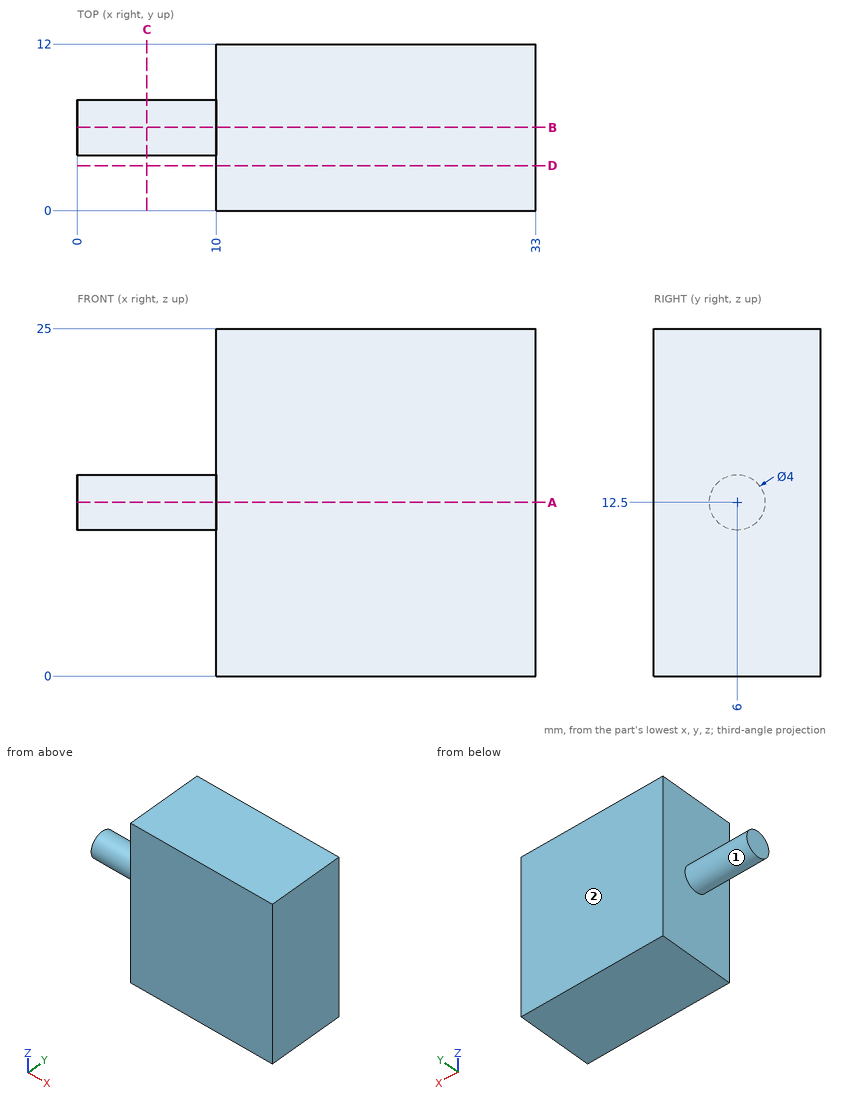
Geometry: see drawing. Coordinates: mm, zero at the bounding-box minimum. A direction names the side the tool comes from. Round coordinates to 2 decimals unless told otherwise and drop trailing zeros. Write each loop counter-clockwise with the first axis right and the second up, starting at its lowest first coordinate (ties: lowest second). Pieces come first, ordered by that corner, then holes. Notation, with made-up numbers: (83, 51) -> (98, 51) arc R25 cw to (98, 90) -> close; hole circle Ø5 at (-30, -10.5). An arc over 180 degrees is marked (long way). Answer as CSV lines item,"result".
1. Section C-C (x = 5). Return the cut outline in (y, z), plus the area to 3 significant figures.
Geometry says:
outline,"circle Ø4 at (6, 12.5)"
area,"12.6 mm^2"
2. Section A-A (z = 12.5). Return the cut outline in (x, y), plus the area to 3 significant figures.
Geometry says:
outline,"(0, 4) -> (10, 4) -> (10, 0) -> (33, 0) -> (33, 12) -> (10, 12) -> (10, 8) -> (0, 8) -> close"
area,"316 mm^2"
3. Section B-B (y = 6). Return the cut outline in (x, z), plus the area to 3 significant figures.
Geometry says:
outline,"(0, 10.5) -> (10, 10.5) -> (10, 0) -> (33, 0) -> (33, 25) -> (10, 25) -> (10, 14.5) -> (0, 14.5) -> close"
area,"615 mm^2"
4. Ray query, L1, parallel to X at y = 9, z = 19. Return the intervals inside material, ascending. Write a range as [from, to].
Geometry says:
L1,"x = [10, 33]"
5. Section D-D (y = 3.25). Return the cut outline in (x, z), plus the area to 3 significant figures.
Geometry says:
outline,"(10, 0) -> (33, 0) -> (33, 25) -> (10, 25) -> close"
area,"575 mm^2"
6. Contact query for flat-ended pins moving along their axis: P1, Ø8, axis at x = 10, z = 10.5, coming from the -Y side; P2, Ø1, axis at y = 4.5, z = 22, coming from the -X side. Output: stop coordinate, or through.
Geometry says:
P1,"stops at y = 0"
P2,"stops at x = 10"
7. Reachability of the marked faces 1 and 2 from +Z, -Z, +X, -X, +Y, -Y: full face, straight path, thin tool, end or side. Return the list, or none.
Geometry says:
face 1,"-X"
face 2,"+Z, -Z, +X, -X, +Y"
